CAD build for the part. Positions are in the model's coordinates, mm. A direction names the side the tool comes from. Give positions to 0.01 mm unless a question says otherwise; leave off trailing zeros. Loops run counter-clockwise (first coordinate to the right, second up) from the corner with the lowest first, then second, coordinate; pieces in that order, holes last. Notation, with made-up numbers: (28.25, -24) -> (45.25, -24) arc R19 ccw to (45.25, -5) -> close; hole circle Ø8 at (72, 2). An arc over 180 degrees is marked (long way). Use one line per item in the form item = value.
```python
from build123d import *

# Parameters (mm, degrees)
SKETCH1_W           = 220
SKETCH1_H           = 180
SKETCH1_R           = 1.55
BOSS_EXTRUDE1_DEPTH = 1.5
SKETCH_1_R          = 1
SKETCH_1_R_2        = 2
SKETCH_1_W          = 27.5
SKETCH_1_H          = 1
CUT_EXTRUDE_1_DEPTH = 2.5
SKETCH3_W           = 6.5
SKETCH3_H           = 14
BOSS_EXTRUDE2_DEPTH = 11


with BuildPart() as part:
    # Sketch1 → Boss-Extrude1 (new body)
    with BuildSketch(Plane(origin=(0, 0, 0), x_dir=(1, 0, 0), z_dir=(0, 1, 0))):
        with Locations((110, 90)):
            Rectangle(SKETCH1_W, SKETCH1_H)
        with Locations((70, 177)):
            Circle(SKETCH1_R, mode=Mode.SUBTRACT)
        with Locations((140, 177)):
            Circle(SKETCH1_R, mode=Mode.SUBTRACT)
        with Locations((30, 150)):
            Circle(SKETCH1_R, mode=Mode.SUBTRACT)
        with Locations((30, 65)):
            Circle(SKETCH1_R, mode=Mode.SUBTRACT)
        with Locations((217, 40)):
            Circle(SKETCH1_R, mode=Mode.SUBTRACT)
        with Locations((217, 135)):
            Circle(SKETCH1_R, mode=Mode.SUBTRACT)
        with Locations((70, 3)):
            Circle(SKETCH1_R, mode=Mode.SUBTRACT)
        with Locations((150, 3)):
            Circle(SKETCH1_R, mode=Mode.SUBTRACT)
        with Locations((123, 79)):
            Circle(SKETCH1_R, mode=Mode.SUBTRACT)
    extrude(amount=BOSS_EXTRUDE1_DEPTH)

    # Эскиз1 → Вырез-Вытянуть1 (cut, through all)
    with BuildSketch(Plane(origin=(0, 1.5, 0), x_dir=(1, 0, 0), z_dir=(0, 1, 0))):
        with Locations((187, 83)):
            Circle(SKETCH_1_R)
        with Locations((187, 97)):
            Circle(SKETCH_1_R)
        with Locations((199.6, 79.3)):
            Circle(SKETCH_1_R_2)
        with Locations((199.6, 100.7)):
            Circle(SKETCH_1_R_2)
        with Locations((174.4, 79.3)):
            Circle(SKETCH_1_R_2)
        with Locations((187, 75.75)):
            Rectangle(SKETCH_1_W, SKETCH_1_H)
        with Locations((187, 104.25)):
            Rectangle(SKETCH_1_W, SKETCH_1_H)
    extrude(amount=-CUT_EXTRUDE_1_DEPTH, mode=Mode.SUBTRACT)

    # Sketch3 → Boss-Extrude2 (add)
    with BuildSketch(Plane(origin=(0, 1.5, 0), x_dir=(1, 0, 0), z_dir=(0, 1, 0))):
        with Locations((202.85, 90.5)):
            Rectangle(SKETCH3_W, SKETCH3_H)
    extrude(amount=BOSS_EXTRUDE2_DEPTH)


solid = part.part
```
1. Drill centre lines: line 1 (Z direction, x = 70, y = 0.7); line 2 (X direction, y = 1.1, z = -79.3); line 3 (Z direction, x = 187, y = 0.65). Where is each one in solid material? Low to high.
Result sheet:
line_1 = -180 to -178.55, -175.45 to -4.55, -1.45 to 0
line_2 = 0 to 121.48, 124.52 to 172.4, 176.4 to 197.6, 201.6 to 220
line_3 = -180 to -104.75, -103.75 to -98, -96 to -84, -82 to -76.25, -75.25 to 0
2. Drop flat-ended pins along their axis: P1, Ø1.5, axis at y = 8.5, z = -88.5, coming from the -X side; P2, Ø6.5, axis at x = 174.4, z = -79.3, coming from the -Y side; P3, Ø4, axis at x = 161, z = -122, coming from the +Y side; P4, Ø5.5, axis at y = 8.5, z = -93.5, coming from the +X side. Give the stop position or say it passes through.
Result sheet:
P1 = 199.6
P2 = 0
P3 = 1.5
P4 = 206.1
3. Tool access for faces 1 (the flat face through (199.6, 7, -90)), 2 (the flat face through (206.1, 7, -90)), 3 (the flat face through (203, 7, -83.5)), 4 (the flat face through (203, 7, -97.5)): list every direction of +Z, -Z, +X, -X, +Y, -Y with a clear straight run to the whole face (end or side of a thin tool).
Result sheet:
face_1 = +Z, -Z, -X, +Y
face_2 = +Z, -Z, +X, +Y
face_3 = +Z, +X, -X, +Y
face_4 = -Z, +X, -X, +Y
4. Cut at A-A, the plane y = 5.5. Write the cut outline in (x, z), then the cut area to 3 significant figures.
Result sheet:
outline = (199.6, -97.5) -> (206.1, -97.5) -> (206.1, -83.5) -> (199.6, -83.5) -> close
area = 91.0 mm^2
5. Cut at B-B, the plane z = -126. Write the cut outline in (x, y), then the cut area to 3 significant figures.
Result sheet:
outline = (0, 0) -> (220, 0) -> (220, 1.5) -> (0, 1.5) -> close
area = 330 mm^2
